from build123d import *

# Parameters (mm, degrees)
EXTRUDE_1_DEPTH  = 0.5
SKETCH_2_R       = 0.4
EXTRUDE_3_DEPTH  = 0.5
SKETCH_3_R       = 0.4
EXTRUDE_12_DEPTH = 0.5


with BuildPart() as part:
    # Эскиз1 → Вытянуть1 (new body)
    with BuildSketch(Plane.XY):
        with BuildLine():
            Line((0, 11.5), (0, -11.5))
            ThreePointArc((0, -11.5), (-0.530330086, -11.40312152), (-0.992156742, -11.125))
            Line((-0.992156742, -11.125), (-5.95294045, -6.75))
            ThreePointArc((-5.95294045, -6.75), (-9, 0), (-5.95294045, 6.75))
            Line((-5.95294045, 6.75), (-0.992156742, 11.125))
            ThreePointArc((-0.992156742, 11.125), (-0.530330086, 11.40312152), (0, 11.5))
        make_face()
    extrude(amount=EXTRUDE_1_DEPTH)

    # Эскиз2 → Вытянуть3 (add)
    with BuildSketch(Plane.XY.offset(0.5)):
        with BuildLine():
            Line((-3.395751311, 12.338562172), (-1.742156742, 10.463562172))
            Line((-1.742156742, 10.463562172), (-3.242156742, 9.140686517))
            Line((-3.242156742, 9.140686517), (-4.895751311, 11.015686517))
            ThreePointArc((-4.895751311, 11.015686517), (-4.807189139, 12.427124344), (-3.395751311, 12.338562172))
        make_face()
        with Locations((-4.145751311, 11.677124344)):
            Circle(SKETCH_2_R, mode=Mode.SUBTRACT)
    extrude(amount=-EXTRUDE_3_DEPTH)

    # Эскиз3 → Вытянуть12 (add)
    with BuildSketch(Plane(origin=(0, 0, 0), x_dir=(-1, 0, 0), z_dir=(0, 0, -1))):
        with BuildLine():
            Line((7.145751311, 9.031373033), (5.492156742, 7.156373033))
            Line((5.492156742, 7.156373033), (2.144002144, -10.109167839))
            Line((2.144002144, -10.109167839), (3.797596713, -11.984167839))
            ThreePointArc((3.797596713, -11.984167839), (5.209034541, -12.072730011), (5.297596713, -10.661292183))
            Line((5.297596713, -10.661292183), (3.644002144, -8.786292183))
            Line((3.644002144, -8.786292183), (5.894002144, -6.8019787))
            Line((5.894002144, -6.8019787), (7.547596713, -8.6769787))
            ThreePointArc((7.547596713, -8.6769787), (8.959034541, -8.765540872), (9.047596713, -7.354103045))
            Line((9.047596713, -7.354103045), (7.061797178, -5.10241802))
            Line((7.061797178, -5.10241802), (7.50995229, -3.016480181))
            Line((7.50995229, -3.016480181), (10.959544642, -3.757610821))
            ThreePointArc((10.959544642, -3.757610821), (12.14728738, -2.989973414), (11.379649973, -1.802230676))
            Line((11.379649973, -1.802230676), (8.149841538, -1.108319701))
            Line((8.149841538, -1.108319701), (8.688125789, 1.397124189))
            Line((8.688125789, 1.397124189), (11.36395596, 2.295342711))
            ThreePointArc((11.36395596, 2.295342711), (11.993742241, 3.561584883), (10.727500069, 4.191371165))
            Line((10.727500069, 4.191371165), (8.034608294, 3.28742543))
            Line((8.034608294, 3.28742543), (6.559673056, 5.343106973))
            Line((6.559673056, 5.343106973), (8.645751311, 7.708497378))
            ThreePointArc((8.645751311, 7.708497378), (8.557189139, 9.119935206), (7.145751311, 9.031373033))
        make_face()
        with Locations((7.895751311, 8.369935206)):
            Circle(SKETCH_3_R, mode=Mode.SUBTRACT)
        with Locations((11.045728014, 3.243356938)):
            Circle(SKETCH_3_R, mode=Mode.SUBTRACT)
        with Locations((11.169597308, -2.779920749)):
            Circle(SKETCH_3_R, mode=Mode.SUBTRACT)
        with Locations((8.297596713, -8.015540872)):
            Circle(SKETCH_3_R, mode=Mode.SUBTRACT)
        with Locations((4.547596713, -11.322730011)):
            Circle(SKETCH_3_R, mode=Mode.SUBTRACT)
    extrude(amount=-EXTRUDE_12_DEPTH)


solid = part.part
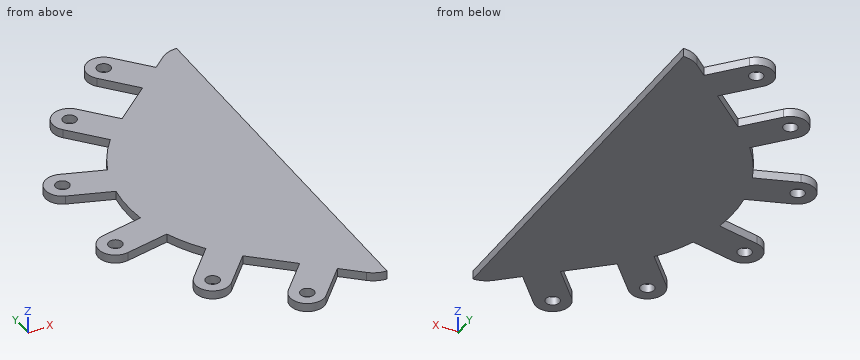
Verification items for the finished model (mm, model axes). Round coordinates to 2 decimals unless told otherwise and drop trailing zeros. Write each loop counter-clockwise with the first axis right and the second up, starting at its lowest first coordinate (ties: lowest second). Pieces come first, ordered by that corner, then holes.
(1) Section check D-D (y = -0.75). Enter the section's corners in (x, z), plus the area to 3 significant figures.
Returned:
outline: (-8.97, 0) - (0, 0) - (0, 0.5) - (-8.97, 0.5) - close
area: 4.48 mm2
(2) Section check A-A (y = 10.75). Enter the section's corners in (x, z).
Returned:
outline: (-4.66, 0) - (-1.99, 0) - (-1.99, 0.5) - (-4.66, 0.5) - close; (-1.42, 0) - (0, 0) - (0, 0.5) - (-1.42, 0.5) - close
(3) Material ranges on line 1 (Y direction, x = -4, z = 0.3); line 2 (X direction, y = 6.25, z = 0.2); line 3 (X direction, y = -3, z = 0.05), recorded low to high.
Returned:
line 1: y = -12.16 to -9.19, -8.47 to 8.47, 10 to 11.3, 12.05 to 12.67
line 2: x = -7.36 to 0
line 3: x = -12.15 to -11.5, -10.84 to 0
(4) Section check C-C (z = 0.1). Give the number of separate pieces and of enclosed holes in the cut face, plus the area to 3 significant figures.
Returned:
separate pieces: 1
enclosed holes: 6
area: 176 mm2
(5) Section check B-B (x = -10). Enter the section's corners in (y, z).
Returned:
outline: (-3.55, 0) - (-1.51, 0) - (-1.51, 0.5) - (-3.55, 0.5) - close; (1.84, 0) - (3.95, 0) - (3.95, 0.5) - (1.84, 0.5) - close
